Drawing for the job (mm, zero at the part's lowest x, y, z). A direction names the side the tool comes from. Coordinates: 2 decimals unless noted, no trailing zeros. Order: outer loops, then holes, each group sorted by start corner. A loop starts at its lowest first (then second) coordinate and runs counter-clockwise, first axis right, second up. Notation, with made-up numbers: (-30.75, 74) -> (19.25, 74) arc R15 cw to (19.25, 96) -> close; hole circle Ø9 at (69.25, 22.5). An arc over 180 degrees is marked (long way). Write each question's results on one line, items separated by ' | '.
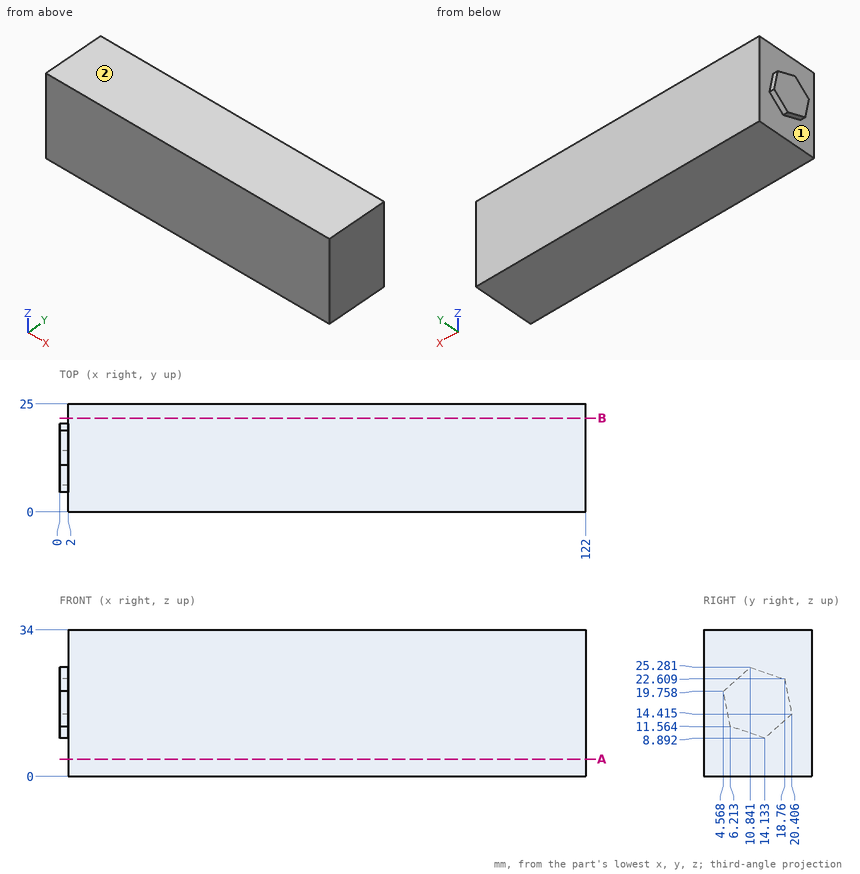
Item 1: Slice it at A-A, the plane z = 4. List the corners of the cut face in (x, y).
Answer:
outline: (2, 0) -> (122, 0) -> (122, 25) -> (2, 25) -> close
Item 2: Slice it at B-B, the plane y = 21.75. List the corners of the cut face in (x, z), and give its area (3 significant figures).
Answer:
outline: (2, 0) -> (122, 0) -> (122, 34) -> (2, 34) -> close | area: 4,080 mm^2
Item 3: Pin check, flat tip, straight feed: pin 1 (1.5 mm diameter, centred on x = 108.5, y = 9.5, fed in from -Z). Stop position of the tip, or through.
Answer:
pin 1: stops at z = 0
Item 4: Tool access for the marked faces 1 and 2: list every direction of +Z, -Z, +X, -X, +Y, -Y with a clear straight run to the whole face (end or side of a thin tool).
Answer:
face 1: -X | face 2: +Z, +X, -X, +Y, -Y
Item 5: Drill centre line: line 1 (X direction, y = 23.5, z = 3.5). Where is it in solid material? Low to high. Write a range as from..to.
Answer:
line 1: x = 2..122
